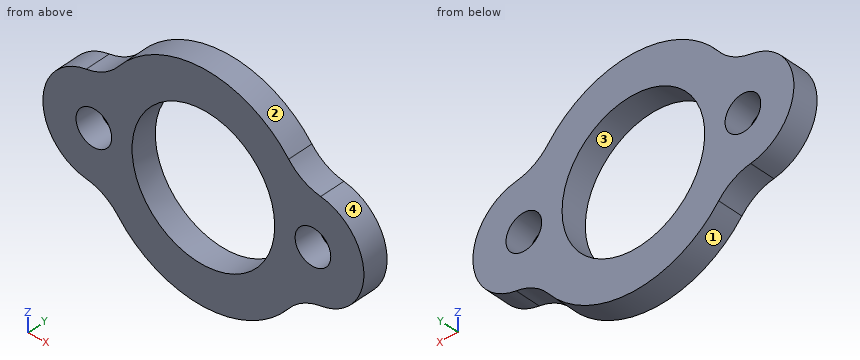
from build123d import *

# Parameters (mm, degrees)
BOSS_EXTRUDE2_OUTLINE_R   = 3.5
BOSS_EXTRUDE2_OUTLINE_R_2 = 14
BOSS_EXTRUDE2_DEPTH       = 5
FILLET2_R                 = 10


# Read off the part's stored shape, not the designer's step: Boss-Extrude2
with BuildPart() as part:
    # Boss-Extrude2 outline → Boss-Extrude2 (new body)
    with BuildSketch(Plane(origin=(0, 0, 0), x_dir=(1, 0, 0), z_dir=(0, 1, 0))):
        with BuildLine():
            ThreePointArc((19.174418605, 9.725824961), (0, 21.5), (-19.174418605, 9.725824961))
            ThreePointArc((-19.174418605, 9.725824961), (-31.5, 0), (-19.174418605, -9.725824961))
            ThreePointArc((-19.174418605, -9.725824961), (0, -21.5), (19.174418605, -9.725824961))
            ThreePointArc((19.174418605, -9.725824961), (31.5, 0), (19.174418605, 9.725824961))
        make_face()
        with Locations((-21.5, 0)):
            Circle(BOSS_EXTRUDE2_OUTLINE_R, mode=Mode.SUBTRACT)
        Circle(BOSS_EXTRUDE2_OUTLINE_R_2, mode=Mode.SUBTRACT)
        with Locations((21.5, 0)):
            Circle(BOSS_EXTRUDE2_OUTLINE_R, mode=Mode.SUBTRACT)
    extrude(amount=BOSS_EXTRUDE2_DEPTH)

    # Fillet2
    fillet2_edges = [part.edges().sort_by_distance(p)[0] for p in [
        (19.174418605, 2.5, -9.725824961),
        (19.174418605, 2.5, 9.725824961),
        (-19.174418605, 2.5, 9.725824961),
        (-19.174418605, 2.5, -9.725824961),
    ]]
    fillet(fillet2_edges, radius=FILLET2_R)


solid = part.part
Part model, mm, in its own coordinate system. Face numbers are marked on the shaded views. Coordinates: 2 decimals unless noted, no trailing zeros. Loops run counter-clockwise (first coordinate to the right, second up) from the corner with the lowest first, then second, coordinate; pieces in that order, holes last. Notation, with made-up numbers: M -1,17.5 L 48,17.5 A10 cw 48,25.5 Z; hole C -37.75,77.5 d11. An arc over 180 degrees is marked long. Use a Markdown table: item, result. Add a question column.
Q1. Probe L1, parallel to X at y = 1.5, z = 0; L2, parallel to Z at x = 21.5, y = 2.95; L3, parallel to Z at x = -24, y = 2.9. List the from-to ranges inside material, lowest first.
Q2. Cut at D-D (y = 3.6). Give the number of separate pieces and of enclosed holes in the cut face, and give its area (3 significant figures).
Q3. Cut at B-B (z = 0). Write the cut outline in (x, y).
Q4. Mould opens along Z. For the marked faces 1, 2, 3 and 4 say: +Z half, -Z half, draft (parallel to the pull), parting line (faces both ways), or undercut.
Q5. Pin check, flat tips, straight feed: P1, Ø2, axis at x = 16, z = 16, coming from the -Y side (3 decimals); P2, Ø2, axis at x = -22.5, y = 1.5, coming from the +Z side. Stop position of each tip, or through.
Q6. Cut at A-A (x = 0). Write the cut outline in (y, z), and give its area (3 significant figures).
Q7. Cut at C-C (z = 4.5). Write the cut outline in (x, y).
Worked out:
| question | item | result |
|---|---|---|
| 1 | L1 | x = -31.5 to -25, -18 to -14, 14 to 18, 25 to 31.5 |
| 1 | L2 | z = -10.24 to -3.5, 3.5 to 10.24 |
| 1 | L3 | z = -9.68 to -2.45, 2.45 to 9.68 |
| 2 | separate pieces | 1 |
| 2 | enclosed holes | 3 |
| 2 | area | 1,120 mm2 |
| 3 | outline | M -31.5,0 L -25,0 L -25,5 L -31.5,5 Z; M -18,0 L -14,0 L -14,5 L -18,5 Z; M 14,0 L 18,0 L 18,5 L 14,5 Z; M 25,0 L 31.5,0 L 31.5,5 L 25,5 Z |
| 4 | face 1 | -Z half |
| 4 | face 2 | +Z half |
| 4 | face 3 | undercut |
| 4 | face 4 | parting line |
| 5 | P1 | passes through |
| 5 | P2 | stops at z = 10.24 |
| 6 | outline | M 0,-21.5 L 5,-21.5 L 5,-14 L 0,-14 Z; M 0,14 L 5,14 L 5,21.5 L 0,21.5 Z |
| 6 | area | 75.0 mm2 |
| 7 | outline | M -30.43,0 L -13.26,0 L -13.26,5 L -30.43,5 Z; M 13.26,0 L 30.43,0 L 30.43,5 L 13.26,5 Z |
